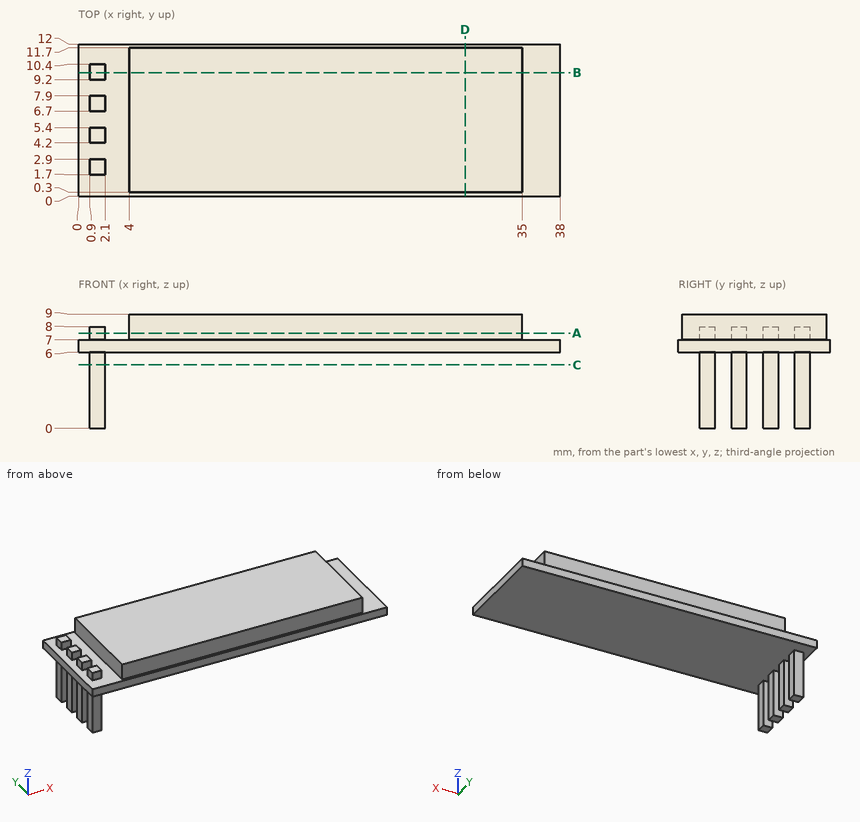
Job drawing, mm, ordinate dimensions from the low corner. One solid piece. Give positions to 0.01 mm unless a question says otherwise; leave off trailing zeros. Loops run counter-clockwise (first coordinate to the right, second up) from the corner with the lowest first, then second, coordinate; pieces in that order, holes last. Notation, with made-up numbers: (-19, 56.5) -> (26, 56.5) arc R10 ccw to (26, 73.5) -> close; hole circle Ø9 at (-33.5, -36.5). An arc over 180 degrees is marked (long way). Use a Markdown table: item, result. Add a question column.
(1) Slice it at B-B on y = 9.75. List the corners of the cut face in (x, z).
(2) Drop flat-ended pins along their axis: pin 1 Ø0.6 at (x, z) = (15, 8) entering from -Y; pin 2 Ø0.8 at (x, z) = (1.5, 7.5) entering from +Y; pin 3 Ø4 at (y, z) = (3, 3) entering from -X. Give the stop position or say it passes through.
(3) Slice it at A-A on z = 7.5. List the corners of the cut face in (x, y), and give its area (3 significant figures).
(4) Slice it at C-C on z = 5. List the corners of the cut face in (x, y), and give its area (3 significant figures).
(5) Wall check: line 1 along X through (y, z) = (4.25, 7.5); line 2 along Z through (x, y) = (18.5, 9); line 3 along X through (y, z) = (4, 8). Give the ranges that are in metal, low to high.
(6) Slice it at D-D on x = 30.5. List the corners of the cut face in (y, z), and give its area (3 significant figures).
Filled sheet:
| question | item | result |
|---|---|---|
| 1 | outline | (0, 6) -> (0.9, 6) -> (0.9, 0) -> (2.1, 0) -> (2.1, 6) -> (38, 6) -> (38, 7) -> (35, 7) -> (35, 9) -> (4, 9) -> (4, 7) -> (2.1, 7) -> (2.1, 8) -> (0.9, 8) -> (0.9, 7) -> (0, 7) -> close |
| 2 | pin 1 | y = 0.3 |
| 2 | pin 2 | y = 10.4 |
| 2 | pin 3 | x = 0.9 |
| 3 | outline | (0.9, 1.7) -> (2.1, 1.7) -> (2.1, 2.9) -> (0.9, 2.9) -> close; (0.9, 4.2) -> (2.1, 4.2) -> (2.1, 5.4) -> (0.9, 5.4) -> close; (0.9, 6.7) -> (2.1, 6.7) -> (2.1, 7.9) -> (0.9, 7.9) -> close; (0.9, 9.2) -> (2.1, 9.2) -> (2.1, 10.4) -> (0.9, 10.4) -> close; (4, 0.3) -> (35, 0.3) -> (35, 11.7) -> (4, 11.7) -> close |
| 3 | area | 359 mm2 |
| 4 | outline | (0.9, 1.7) -> (2.1, 1.7) -> (2.1, 2.9) -> (0.9, 2.9) -> close; (0.9, 4.2) -> (2.1, 4.2) -> (2.1, 5.4) -> (0.9, 5.4) -> close; (0.9, 6.7) -> (2.1, 6.7) -> (2.1, 7.9) -> (0.9, 7.9) -> close; (0.9, 9.2) -> (2.1, 9.2) -> (2.1, 10.4) -> (0.9, 10.4) -> close |
| 4 | area | 5.76 mm2 |
| 5 | line 1 | 0.9 to 2.1, 4 to 35 |
| 5 | line 2 | 6 to 9 |
| 5 | line 3 | 4 to 35 |
| 6 | outline | (0, 6) -> (12, 6) -> (12, 7) -> (11.7, 7) -> (11.7, 9) -> (0.3, 9) -> (0.3, 7) -> (0, 7) -> close |
| 6 | area | 34.8 mm2 |
